Source: CAD feature listing. Evaluate the final solid. Frame: model axes, mm. Face numbers are marked on the shaded views. A direction names the side the tool comes from. Round coordinates to 2 decimals unless told otherwise and drop trailing zeros. Loops run counter-clockwise (first coordinate to the right, second up) from the corner with the lowest first, then second, coordinate; pieces in that order, holes last. Notation, with made-up numbers: (-35.75, -8) - (15.25, -8) arc R8 ccw to (15.25, 7) - close; hole circle Ø6 at (-23, -10.75). An arc over 180 degrees is marked (long way). Write item = value, one per line. Start each with the question number.
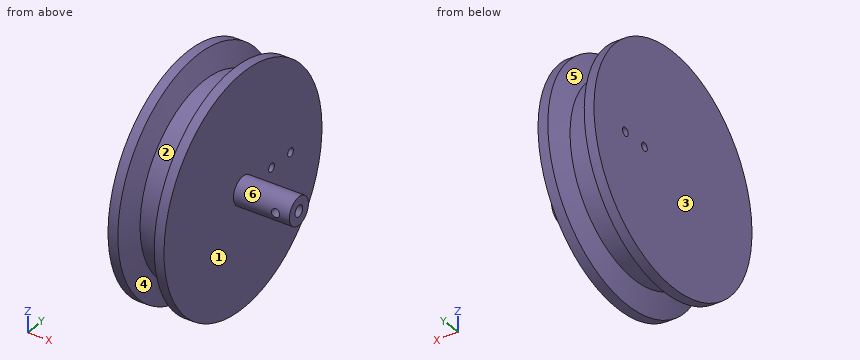
Autodesk Inventor part; units mm, degrees
ref_plane "РабПлоскость1" through (0, 5, 0) normal (0, 1, 0) x (-1, 0, 0)
ref_plane "РабПлоскость2" through (-10, 0, 0) normal (-1, 0, 0) x (0, 0, 1)
ref_plane "YZ Plane" through (0, 0, 0) normal (1, 0, 0) x (0, 1, 0)
sketch "Эскиз1" plane through (0, 0, 0) normal (0, 1, 0) x (-1, 0, 0)
  line L0 (0, 0) -> (20, 0)
  line L1 (20, 0) -> (20, 41.5)
  line L2 (20, 41.5) -> (0, 41.5)
  line L3 (0, 41.5) -> (0, 0)
  line L4 (20, 41.5) -> (14, 41.5)
  line L5 (14, 41.5) -> (14, 33.5)
  line L6 (14, 33.5) -> (6, 33.5)
  line L7 (6, 33.5) -> (6, 41.5)
  line L8 (10, 33.5) -> (10, 41.5)
  line L9 (10, 41.5) -> (3.5, 41.5)
  line L10 (3.5, 41.5) -> (6, 33.5)
  line L11 (10, 41.5) -> (16.5, 41.5)
  line L12 (16.5, 41.5) -> (14, 33.5)
  dimension "d0" = 20
  dimension "d1" = 41.5
  dimension "d2" = 6
  dimension "d3" = 8
  dimension "d4" = 8
  dimension "d38" = 6.5
  dimension "d39" = 6.5
revolve "Вращение1" add sketch "Эскиз1" angle 360 about axis through (0, 0, 0) along (-1, 0, 0) contours L3 L2 L10 L6 L12 L1 L0
sketch "Эскиз2" plane through (0, 0, 0) normal (1, 0, 0) x (0, 0, -1)
  circle A0 centre (0, 0) radius 5
  dimension "d6" = 10
extrude "Выдавливание1" add sketch "Эскиз2" along normal blind 20
sketch "Эскиз3" plane through (20, 0, 0) normal (1, 0, 0) x (0, 0, -1)
  circle A0 centre (0, 0) radius 2
  dimension "d9" = 4
extrude "Выдавливание2" cut sketch "Эскиз3" against normal blind 20
sketch "Эскиз4" plane through (0, 0, 0) normal (1, 0, 0) x (0, 0, -1)
  circle A0 centre (0, 0) radius 5
  point P0 (0, 5)
ref_plane "РабПлоскость1" through (0, 5, 0) normal (0, 1, 0) x (-1, 0, 0)
sketch "Эскиз5" plane through (0, 5, 0) normal (0, 1, 0) x (-1, 0, 0)
  line L0 (0, 0) -> (-15, 0)
  circle A0 centre (-15, 0) radius 1.5
  dimension "d18" = 15
  dimension "d19" = 3
extrude "Выдавливание3" cut sketch "Эскиз5" against normal blind 58
thread "Резьба1"
ref_plane "РабПлоскость2" through (-10, 0, 0) normal (-1, 0, 0) x (0, 0, 1)
sketch "Эскиз6" plane through (0, 0, 0) normal (1, 0, 0) x (0, 0, -1)
  circle A0 centre (0, 0) radius 5
  line L0 (0, 0) -> (0, 25)
  circle A1 centre (0, 25) radius 1.5
  line L1 (0, 0) -> (0, 15)
  circle A2 centre (0, 15) radius 1.5
  dimension "d28" = 25
  dimension "d29" = 3
  dimension "d42" = 15
  dimension "d43" = 3
extrude "Выдавливание4" cut sketch "Эскиз6" against normal blind 59.75 contours A1 | A2 L0 | L0 A2
thread "Резьба2"
thread "Резьба3"
properties part number "17701729.303661.005"
(1) Cut plane B-B (y = 0). Output: boundary loops of the cut face in (x, z), and give its area (3 significant figures).
(2) Mould query, pull axis X, two halves, no side actions, for the marked faces 1, 2, 3 and 4. Classes: +X half, -X half, draft (parallel to the pull), parting line (faces both ways), or undercut.
(3) Cut plane C-C (z = 0). State how many separate pieces and enclosed holes the cut face has, and give its area (3 significant figures).
(4) Pin query (flat end, axial travel): P1, Ø5, axis at y = -24.5, z = -8.5, coming from the +X side; P2, Ø1.8, axis at y = 25, z = 0, coming from the -X side; P3, Ø2, axis at x = 6.5, z = 0.5, coming from the -Y side; P4, Ø5, axis at x = 15, z = 0, coming from the +Y side. Return the tip coordinate at first contact, or that it passes through.
(5) Access query for the marked faces 5 and 6. Directions: +Z, -Z, +X, -X, +Y, -Y. A direction counts if a zero-diameter tool reaches every point of the face in a straight line with its end or side. Return the directions, or none.
(6) Cut plane A-A (x = 14.5). Output: boundary loops of the cut face in (y, z), and give its area (3 significant figures).
(7) Cut plane D-D (x = -2.5). Output: boundary loops of the cut face in (y, z), and give its area (3 significant figures).
(8) Material intervals for line 1 along X through (y, z) = (-3.85, 0); line 2 along Y through (x, z) = (9.75, 0); line 3 along X through (y, z) = (-17.5, -1.5), sorted ascending. Write a range as from..to.
Solution:
q1.outline = (-20, -41.5) - (-16.5, -41.5) - (-14, -33.5) - (-6, -33.5) - (-3.5, -41.5) - (0, -41.5) - (0, -5) - (20, -5) - (20, -2) - (0, -2) - (0, 2) - (20, 2) - (20, 5) - (0, 5) - (0, 41.5) - (-3.5, 41.5) - (-6, 33.5) - (-14, 33.5) - (-16.5, 41.5) - (-20, 41.5) - close
q1.area = 1,610 mm^2
q2.face_1 = +X half
q2.face_2 = undercut
q2.face_3 = -X half
q2.face_4 = undercut
q3.separate_pieces = 5
q3.enclosed_holes = 0
q3.area = 1,470 mm^2
q4.P1 = 0
q4.P2 = through
q4.P3 = -5
q4.P4 = 5
q5.face_5 = none
q5.face_6 = +X
q6.outline = (-4.8, -1.41) arc R5 ccw to (4.8, -1.41) - (1.41, -1.41) arc R2 cw to (-1.41, -1.41) - close; (-4.8, 1.41) - (-1.41, 1.41) arc R2 cw to (1.41, 1.41) - (4.8, 1.41) arc R5 ccw to start
q6.area = 48.4 mm^2
q7.outline = circle Ø83 at (0, 0); hole circle Ø3 at (15, 0); hole circle Ø3 at (25, 0)
q7.area = 5,400 mm^2
q8.line_1 = -20..13.5, 16.5..20
q8.line_2 = -5..-2, 2..5
q8.line_3 = -20..0
